from build123d import *

# Parameters (mm, degrees)
BOSS_EXTRUDE1_DEPTH     = 4
SKETCH2_R               = 2.5
CUT_EXTRUDE1_DEPTH      = 64.702725576
CUT_EXTRUDE2_DEPTH      = 1.25
SKETCH4_R               = 3.75
SKETCH4_R_2             = 2.5
BOSS_EXTRUDE2_DEPTH     = 1.25
CUT_EXTRUDE8_DEPTH      = 64.702725576
CUT_EXTRUDE8_DEPTH_BACK = 64.702725576
CUT_EXTRUDE9_DEPTH      = 64.702725576
CUT_EXTRUDE9_DEPTH_BACK = 64.702725576
FILLET5_R               = 1
FILLET6_R               = 1
FILLET7_R               = 1
FILLET8_R               = 1


with BuildPart() as part:
    # Sketch1 → Boss-Extrude1 (new, symmetric)
    with BuildSketch(Plane.XY):
        with BuildLine():
            Line((-35, 0), (35, 0))
            ThreePointArc((35, 0), (41.5, 6.5), (35, 13))
            Line((35, 13), (13.916352203, 13))
            ThreePointArc((13.916352203, 13), (6.053324797, 16.256972593), (2.796352203, 24.12))
            Line((2.796352203, 24.12), (2.796352203, 27.12))
            Line((2.796352203, 27.12), (-7.213647797, 27.12))
            ThreePointArc((-7.213647797, 27.12), (-22.934441841, 13.089935965), (-43.483647797, 17.75))
            Line((-43.483647797, 17.75), (-57.083647797, 17.75))
            Line((-57.083647797, 17.75), (-57.083647797, 12.75))
            Line((-57.083647797, 12.75), (-35, 0))
        make_face()
    extrude(amount=BOSS_EXTRUDE1_DEPTH, both=True)

    # Sketch2 → Cut-Extrude1 (cut, through all)
    with BuildSketch(Plane(origin=(0, 0, -4), x_dir=(-1, 0, 0), z_dir=(0, 0, -1))):
        with Locations((-35, 6.5)):
            Circle(SKETCH2_R)
        with Locations((-5, 6.5)):
            Circle(SKETCH2_R)
    extrude(amount=-CUT_EXTRUDE1_DEPTH, mode=Mode.SUBTRACT)

    # Sketch3 → Cut-Extrude2 (cut)
    with BuildSketch(Plane.XY.offset(4)):
        with BuildLine():
            Line((-44.195256898, 15.75), (-55.083647797, 15.75))
            Line((-55.083647797, 15.75), (-55.083647797, 13.904700538))
            Line((-55.083647797, 13.904700538), (-34.464101615, 2))
            Line((-34.464101615, 2), (35, 2))
            ThreePointArc((35, 2), (39.5, 6.5), (35, 11))
            Line((35, 11), (13.916352203, 11))
            ThreePointArc((13.916352203, 11), (4.639111234, 14.842759031), (0.796352203, 24.12))
            Line((0.796352203, 24.12), (0.796352203, 25.12))
            Line((0.796352203, 25.12), (-5.880235749, 25.12))
            ThreePointArc((-5.880235749, 25.12), (-22.748609603, 11.074453376), (-44.195256898, 15.75))
        make_face()
    cut_extrude2 = extrude(amount=-CUT_EXTRUDE2_DEPTH, mode=Mode.SUBTRACT)

    # Sketch4 → Boss-Extrude2 (add)
    # profile 1 of 2: a face of its own
    with BuildSketch(Plane.XY.offset(2.75)):
        with Locations((5, 6.5)):
            Circle(SKETCH4_R)
        with Locations(Location((5, 6.5, 0), (0, 0, 180))):
            Circle(SKETCH4_R_2, mode=Mode.SUBTRACT)
    # profile 2 of 2: a face of its own
    with BuildSketch(Plane.XY.offset(2.75)):
        with Locations((35, 6.5)):
            Circle(SKETCH4_R)
        with Locations(Location((35, 6.5, 0), (0, 0, 180))):
            Circle(SKETCH4_R_2, mode=Mode.SUBTRACT)
    boss_extrude2 = extrude(amount=BOSS_EXTRUDE2_DEPTH)

    # Mirror1: Cut-Extrude2, Boss-Extrude2 across plane
    add(cut_extrude2.mirror(Plane.XY), mode=Mode.SUBTRACT)
    add(boss_extrude2.mirror(Plane.XY))

    # Sketch6 → Cut-Extrude8 (cut, two sides: drawn at the far end of the back side and taken through both)
    with BuildSketch(Plane.XY.offset(4).offset(-CUT_EXTRUDE8_DEPTH_BACK)):
        Polygon((-201.988502331, 164.254854535), (-55.483647797, 17.75), (-53.750566679, 16.016918882), (-53.214504533, 16.016918882), (-51.481423415, 17.75), (-49.748342297, 16.016918882), (-49.212280151, 16.016918882), (-47.479199033, 17.75), (-45.746117916, 16.016918882), (-45.21005577, 16.016918882), (-43.476974652, 17.75), (103.027879883, 164.254854535), (103.027879883, 578.633159007), (-201.988502331, 578.633159007), align=None)
    extrude(amount=CUT_EXTRUDE8_DEPTH + CUT_EXTRUDE8_DEPTH_BACK, mode=Mode.SUBTRACT)

    # Sketch9 → Cut-Extrude9 (cut, two sides: drawn at the far end of the back side and taken through both)
    with BuildSketch(Plane.XY.offset(4).offset(-CUT_EXTRUDE9_DEPTH_BACK)):
        Polygon((-3.613647797, 27.12), (-7.213647797, 27.12), (-5.413647797, 25.32), align=None)
        Polygon((-0.013647797, 27.12), (-3.613647797, 27.12), (-1.813647797, 25.32), align=None)
        Polygon((2.796352203, 27.12), (-0.013647797, 27.12), (2.796352203, 24.31), align=None)
    extrude(amount=CUT_EXTRUDE9_DEPTH + CUT_EXTRUDE9_DEPTH_BACK, mode=Mode.SUBTRACT)

    # Fillet5
    fillet5_edges = [part.edges().sort_by_distance(p)[0] for p in [
        (-55.083647797, 15.75, 3.375),
    ]]
    fillet(fillet5_edges, radius=FILLET5_R)

    # Fillet6
    fillet6_edges = [part.edges().sort_by_distance(p)[0] for p in [
        (-44.195256898, 15.75, 3.375),
        (-55.083647797, 13.904700538, 3.375),
    ]]
    fillet(fillet6_edges, radius=FILLET6_R)

    # Fillet7
    fillet7_edges = [part.edges().sort_by_distance(p)[0] for p in [
        (0.796352203, 25.12, 3.375),
        (-34.464101615, 2, 3.375),
        (-5.880235749, 25.12, 3.375),
    ]]
    fillet(fillet7_edges, radius=FILLET7_R - 0.0001)  # a hair under: the kernel refuses the full size

    # Fillet8
    fillet8_edges = [part.edges().sort_by_distance(p)[0] for p in [
        (-55.083647797, 13.904700538, -3.375),
        (-34.464101615, 2, -3.375),
        (-44.195256898, 15.75, -3.375),
        (-55.083647797, 15.75, -3.375),
        (-5.880235749, 25.12, -3.375),
        (0.796352203, 25.12, -3.375),
    ]]
    fillet(fillet8_edges, radius=FILLET8_R - 0.0001)  # a hair under: the kernel refuses the full size


solid = part.part
Model file for the job. Use its own axes, mm. A direction names the side the tool comes from. Give positions to 0.01 mm unless a question says otherwise; leave off trailing zeros. Loops run counter-clockwise (first coordinate to the right, second up) from the corner with the lowest first, then second, coordinate; pieces in that order, holes last.
1) Flat gauge pins, fed straight in: pin 1 Ø1 at (x, z) = (-48.5, 3.5) entering from -Y; pin 2 Ø1 at (x, z) = (-3, -3.5) entering from +Y; pin 3 Ø0.6 at (x, z) = (0.5, 3) entering from +Y. Where does each tip first touch, or does it go through?
2) Pull direction X, two halves, no side cores. Call faces 6 (the cylindrical face through (41.5, 6.4, 0.1)), 7 (the flat face through (-8, 8, 2.75)), 8 (the flat face through (36, 4, 4)): +X half, -X half, draft (parallel to the pull), parting line (faces both ways), or undercut.
3) Saw through at C-C (y = 5.5). Count the separate pieces of the cut face and the enclosed holes in it, plus the area to 3 significant figures.
4) Tool access for faces 1 (the flat face through (0, 0, 0)), 2 (the flat face through (-2.726, 26.233, -0.056)), 3 (the flat face through (1.372, 25.735, -0.056)), 4 (the cylindrical face through (4.742, 14.741, 3.384)), 5 (the flat face through (-44.779, 7.955, -3.384)): list every direction of +Z, -Z, +X, -X, +Y, -Y with a clear straight run to the whole face (end or side of a thin tool).
5) Saw through at D-D (y = 21.25). Write the cut outline in (x, z).
6) Wall check: line 1 (X direction, y = 6.5, z = 2.25); line 2 (X direction, y = 16.75, z = 1.25); line 3 (Y direction, x = 35, z = 1). Give the ranges that are in metal, low to high.
7) Saw through at A-A (x = 5). Write the cut outline in (y, z).
8) Saw through at B-B (z = -0.5). Write the cut outline in (x, y).
Answer block:
1. pin 1: stops at y = 7.51
1. pin 2: stops at y = 27.01
1. pin 3: stops at y = 26.91
2. face 6: +X half
2. face 7: undercut
2. face 8: draft
3. separate pieces: 3
3. enclosed holes: 0
3. area: 451 mm2
4. face 1: +Z, -Z, +X, -X, -Y
4. face 2: +Z, -Z, +Y
4. face 3: +Z, -Z, +X, +Y
4. face 4: +Z
4. face 5: -Z
5. outline: (-10.52, -4) - (-8.05, -4) - (-8.05, -2.75) - (1.11, -2.75) - (1.11, -4) - (3.17, -4) - (3.17, 4) - (1.11, 4) - (1.11, 2.75) - (-8.05, 2.75) - (-8.05, 4) - (-10.52, 4) - close
6. line 1: x = -46.26 to 2.5, 7.5 to 32.5, 37.5 to 41.5
6. line 2: x = -57.08 to -54.48, -52.48 to -50.48, -48.48 to -46.48, -44.48 to -42.2, -15.17 to 5.59
6. line 3: y = 0 to 4, 9 to 13
7. outline: (0, -4) - (2, -4) - (2, -2.75) - (2.75, -2.75) - (2.75, -4) - (4, -4) - (4, 4) - (2.75, 4) - (2.75, 2.75) - (2, 2.75) - (2, 4) - (0, 4) - close; (9, -4) - (10.25, -4) - (10.25, -2.75) - (14.5, -2.75) - (14.5, -4) - (17.48, -4) - (17.48, 4) - (14.5, 4) - (14.5, 2.75) - (10.25, 2.75) - (10.25, 4) - (9, 4) - close
8. outline: (-57.08, 12.75) - (-35, 0) - (35, 0) arc R6.5 ccw to (35, 13) - (13.92, 13) arc R11.12 cw to (2.8, 24.12) - (2.8, 24.31) - (-0.01, 27.12) - (-1.81, 25.32) - (-3.61, 27.12) - (-5.41, 25.32) - (-7.21, 27.12) arc R23 cw to (-43.48, 17.75) - (-45.21, 16.02) - (-45.75, 16.02) - (-47.48, 17.75) - (-49.21, 16.02) - (-49.75, 16.02) - (-51.48, 17.75) - (-53.21, 16.02) - (-53.75, 16.02) - (-55.48, 17.75) - (-57.08, 17.75) - close; hole circle Ø5 at (5, 6.5); hole circle Ø5 at (35, 6.5)
